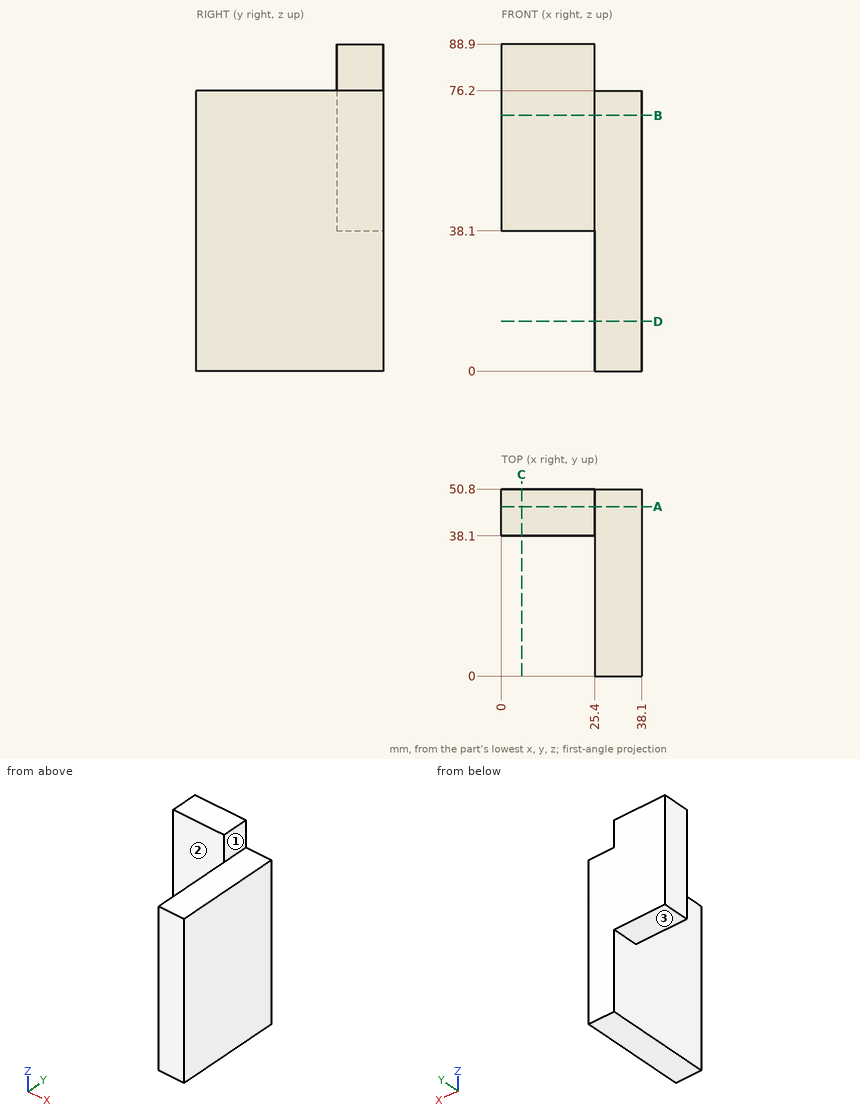
Check sheet for the drawn part. Datum: minimum x, y, z corner. Units: mm. A direction names the side the tool comes from. Round coordinates to 2 decimals unless told otherwise and drop trailing zeros. Loops run counter-clockwise (first coordinate to the right, second up) from the corner with the lowest first, then second, coordinate; pieces in that order, holes last. Notation, with made-up numbers: (17, -31.75) -> (24, -31.75) arc R22 cw to (24, -11.75) -> close; hole circle Ø7 at (73.25, 6.5). An arc over 180 degrees is marked (long way). Put each result on its own line as item: value. Start each with the question number.
1. Scan lines: probe 1 along Y at (x, z) = (17, 74); probe 2 along X at (y, z) = (16, 13); probe 3 along X at (y, z) = (41, 80). Record each from-to range of solid material in increasing order.
2. Section check C-C (x = 5.5). Enter the section's corners in (y, z).
3. Section check B-B (z = 69.5). Enter the section's corners in (x, y), plus the area to 3 significant figures.
4. Access from +Z, -Z, +X, -X, +Y, -Y to the whole of each face (thin tool, end or side, straight path). Record for the marked faces 1, 2 and 3.
5. Section check D-D (z = 13.5). Enter the section's corners in (x, y), plus the area to 3 significant figures.
6. Section check A-A (y = 46). Enter the section's corners in (x, z).
7. Gauge pin test, flat ends, axial feed: pin 1 (4 mm diameter, centred on x = 13, y = 41.5, fed in from -Z); pin 2 (1.5 mm diameter, centred on x = 21.5, z = 72, fed in from -Y); pin 3 (6 mm diameter, centred on y = 21, z = 51, fed in from -X); pin 4 (6 mm diameter, centred on x = 20, z = 24, fed in from +Y). Record the tip position at first contact, or that the pin passes through.
Findings:
1. probe 1: y = 38.1 to 50.8
1. probe 2: x = 25.4 to 38.1
1. probe 3: x = 0 to 25.4
2. outline: (38.1, 38.1) -> (50.8, 38.1) -> (50.8, 88.9) -> (38.1, 88.9) -> close
3. outline: (0, 38.1) -> (25.4, 38.1) -> (25.4, 0) -> (38.1, 0) -> (38.1, 50.8) -> (0, 50.8) -> close
3. area: 968 mm^2
4. face 1: +Z, +X, +Y, -Y
4. face 2: +Z, -Z, -X, -Y
4. face 3: -Z, -X, +Y, -Y
5. outline: (25.4, 0) -> (38.1, 0) -> (38.1, 50.8) -> (25.4, 50.8) -> close
5. area: 645 mm^2
6. outline: (0, 38.1) -> (25.4, 38.1) -> (25.4, 0) -> (38.1, 0) -> (38.1, 76.2) -> (25.4, 76.2) -> (25.4, 88.9) -> (0, 88.9) -> close
7. pin 1: stops at z = 38.1
7. pin 2: stops at y = 38.1
7. pin 3: stops at x = 25.4
7. pin 4: passes through
